Read the model definition and answer for the solid it produces. Units are mm, in the model's axes. A direction names the side the tool comes from. Round coordinates to 2 decimals unless told otherwise and drop trailing zeros. Write each loop counter-clockwise with the first axis right and the second up, starting at its lowest first coordinate (ties: lowest second). Pieces come first, ordered by that corner, then holes.
from build123d import *

# Parameters (mm, degrees)
SKETCH1_R           = 40
SKETCH1_R_2         = 30
SKETCH1_R_3         = 2.625
BOSS_EXTRUDE1_DEPTH = 19


with BuildPart() as part:
    # Sketch1 → Boss-Extrude1 (new body)
    with BuildSketch(Plane.XY):
        Circle(SKETCH1_R)
        Circle(SKETCH1_R_2, mode=Mode.SUBTRACT)
        with Locations((0, 34)):
            Circle(SKETCH1_R_3, mode=Mode.SUBTRACT)
        with Locations((29.444863729, 17)):
            Circle(SKETCH1_R_3, mode=Mode.SUBTRACT)
        with Locations((29.444863729, -17)):
            Circle(SKETCH1_R_3, mode=Mode.SUBTRACT)
        with Locations((0, -34)):
            Circle(SKETCH1_R_3, mode=Mode.SUBTRACT)
        with Locations((-29.444863729, -17)):
            Circle(SKETCH1_R_3, mode=Mode.SUBTRACT)
        with Locations((-29.444863729, 17)):
            Circle(SKETCH1_R_3, mode=Mode.SUBTRACT)
        with BuildLine():
            ThreePointArc((-9.738066572, 36.342959214), (-18.8125, 32.584205817), (-26.604892642, 26.604892642))
            ThreePointArc((-26.604892642, 26.604892642), (-26.604892642, 22.892582041), (-22.892582041, 22.892582041))
            ThreePointArc((-22.892582041, 22.892582041), (-16.1875, 28.037572448), (-8.379266585, 31.271848626))
            ThreePointArc((-8.379266585, 31.271848626), (-6.523111285, 34.486803914), (-9.738066572, 36.342959214))
        make_face(mode=Mode.SUBTRACT)
        with BuildLine():
            ThreePointArc((26.604892642, 26.604892642), (18.8125, 32.584205817), (9.738066572, 36.342959214))
            ThreePointArc((9.738066572, 36.342959214), (6.523111285, 34.486803914), (8.379266585, 31.271848626))
            ThreePointArc((8.379266585, 31.271848626), (16.1875, 28.037572448), (22.892582041, 22.892582041))
            ThreePointArc((22.892582041, 22.892582041), (26.604892642, 22.892582041), (26.604892642, 26.604892642))
        make_face(mode=Mode.SUBTRACT)
        with BuildLine():
            ThreePointArc((36.342959214, -9.738066572), (37.625, 0), (36.342959214, 9.738066572))
            ThreePointArc((36.342959214, 9.738066572), (33.128003927, 11.594221873), (31.271848626, 8.379266585))
            ThreePointArc((31.271848626, 8.379266585), (32.375, 0), (31.271848626, -8.379266585))
            ThreePointArc((31.271848626, -8.379266585), (33.128003927, -11.594221873), (36.342959214, -9.738066572))
        make_face(mode=Mode.SUBTRACT)
        with BuildLine():
            ThreePointArc((9.738066572, -36.342959214), (18.8125, -32.584205817), (26.604892642, -26.604892642))
            ThreePointArc((26.604892642, -26.604892642), (26.604892642, -22.892582041), (22.892582041, -22.892582041))
            ThreePointArc((22.892582041, -22.892582041), (16.1875, -28.037572448), (8.379266585, -31.271848626))
            ThreePointArc((8.379266585, -31.271848626), (6.523111285, -34.486803914), (9.738066572, -36.342959214))
        make_face(mode=Mode.SUBTRACT)
        with BuildLine():
            ThreePointArc((-26.604892642, -26.604892642), (-18.8125, -32.584205817), (-9.738066572, -36.342959214))
            ThreePointArc((-9.738066572, -36.342959214), (-6.523111285, -34.486803914), (-8.379266585, -31.271848626))
            ThreePointArc((-8.379266585, -31.271848626), (-16.1875, -28.037572448), (-22.892582041, -22.892582041))
            ThreePointArc((-22.892582041, -22.892582041), (-26.604892642, -22.892582041), (-26.604892642, -26.604892642))
        make_face(mode=Mode.SUBTRACT)
        with BuildLine():
            ThreePointArc((-36.342959214, 9.738066572), (-37.625, 0), (-36.342959214, -9.738066572))
            ThreePointArc((-36.342959214, -9.738066572), (-33.128003927, -11.594221873), (-31.271848626, -8.379266585))
            ThreePointArc((-31.271848626, -8.379266585), (-32.375, 0), (-31.271848626, 8.379266585))
            ThreePointArc((-31.271848626, 8.379266585), (-33.128003927, 11.594221873), (-36.342959214, 9.738066572))
        make_face(mode=Mode.SUBTRACT)
    extrude(amount=BOSS_EXTRUDE1_DEPTH)


solid = part.part
Q1. Flat-ended cylindrical pins translate along their axes: pin 1 Ø6 at (x, z) = (22.5, 9) entering from +Y; pin 2 Ø3 at (x, z) = (-13, 6.5) entering from -Y; pin 3 Ø8 at (x, z) = (26.5, 6) entering from +Y. Find the tip coordinate at first contact, or state that the pin passes through.
Verdict:
pin 1: stops at y = 34.92
pin 2: stops at y = -38.31
pin 3: stops at y = 33.07
Q2. Section A-A (z = 10) is taken. State how many separate pieces and enclosed holes the cut face has, then the cut area to 3 significant figures.
Verdict:
separate pieces: 1
enclosed holes: 13
area: 1,360 mm2
Q3. Which of the six approach directions +Z, -Z, +X, -X, +Y, -Y give full straight-line access (tool end or side, diameter ignored) to faces 1 (the flat face through (-30, -6, 0)), 2 (the cylindrical face through (-32.375, -0.119, 9.367))?
Verdict:
face 1: -Z, +X, -X, +Y, -Y
face 2: +Z, -Z
Q4. Section B-B (x = 0) is taken. Determine the outline of the cut face in (y, z) (3 decimals), then the cut area to 4 significant figures.
Verdict:
outline: (-40, 0) - (-36.625, 0) - (-36.625, 19) - (-40, 19) - close; (-31.375, 0) - (-30, 0) - (-30, 19) - (-31.375, 19) - close; (30, 0) - (31.375, 0) - (31.375, 19) - (30, 19) - close; (36.625, 0) - (40, 0) - (40, 19) - (36.625, 19) - close
area: 180.5 mm2
Q5. Section C-C (y = -1) is taken. Determine the outline of the cut face in (x, z), then the cut area to 3 significant figures.
Verdict:
outline: (-39.99, 0) - (-37.61, 0) - (-37.61, 19) - (-39.99, 19) - close; (-32.36, 0) - (-29.98, 0) - (-29.98, 19) - (-32.36, 19) - close; (29.98, 0) - (32.36, 0) - (32.36, 19) - (29.98, 19) - close; (37.61, 0) - (39.99, 0) - (39.99, 19) - (37.61, 19) - close
area: 181 mm2
Q6. Straight lines are drawn through the part: probe 1 along Y at (x, z) = (0, 13) (3 decimals); probe 2 along Y at (x, z) = (-21, 15); probe 3 along X at (y, z) = (-26.5, 14.75). For each, find the intervals that lie inside material, in ascending order.
Verdict:
probe 1: y = -40 to -36.625, -31.375 to -30, 30 to 31.375, 36.625 to 40
probe 2: y = -34.04 to -31.22, -24.64 to -21.42, 21.42 to 24.64, 31.22 to 34.04
probe 3: x = -29.96 to -26.7, -18.6 to -14.06, 14.06 to 18.6, 26.7 to 29.96
